For this review, take the finished solid that the model builds, in its own axes (mm). A direction names the side the tool comes from. Coordinates: 2 decimals unless noted, no trailing zeros. Loops run counter-clockwise (first coordinate to the right, second up) from the corner with the lowest first, then second, coordinate; pieces in that order, holes last. Notation, with made-up numbers: (28.25, 87) -> (71.25, 87) arc R13 cw to (71.25, 92) -> close; hole circle Ø9 at (85.5, 73.5). An arc over 180 degrees is marked (long way). One line per item, written item: value.
from build123d import *

# Parameters (mm, degrees)
CROQUIS1_W              = 76.2
CROQUIS1_H              = 76.2
CROQUIS1_W_2            = 66.675
CROQUIS1_H_2            = 66.675
SALIENTE_EXTRUIR1_DEPTH = 950
CORTAR_EXTRUIR1_REACH   = 958.093
CORTAR_EXTRUIR2_DEPTH   = 76.2


with BuildPart() as part:
    # Croquis1 → Saliente-Extruir1 (new body)
    with BuildSketch(Plane(origin=(0, 0, 0), x_dir=(1, 0, 0), z_dir=(0, 1, 0))):
        with Locations((38.1, -38.1)):
            Rectangle(CROQUIS1_W, CROQUIS1_H)
        with Locations((38.1, -38.1)):
            Rectangle(CROQUIS1_W_2, CROQUIS1_H_2, mode=Mode.SUBTRACT)
    extrude(amount=SALIENTE_EXTRUIR1_DEPTH)

    # Cortar-Extruir1: up to this face of the body (flat: up to its plane)
    cortar_extruir1_end = Plane(part.part.faces().sort_by_distance((38.1, 475, 0))[0])
    # Croquis2 → Cortar-Extruir1 (cut, up to the picked face)
    with BuildSketch(Plane.XY.offset(76.2), mode=Mode.PRIVATE) as cortar_extruir1_sk1:
        Polygon((0, 0), (76.2, 17.592156164), (76.2, 0), align=None)
    cortar_extruir1_tool1 = split(extrude(cortar_extruir1_sk1.sketch, amount=-CORTAR_EXTRUIR1_REACH, mode=Mode.PRIVATE), bisect_by=cortar_extruir1_end, keep=Keep.BOTH, mode=Mode.PRIVATE)
    add(cortar_extruir1_tool1.solids().sort_by(Axis((50.8, 5.864052, 76.2), (0, 0, -1)))[0], mode=Mode.SUBTRACT)

    # Croquis3 → Cortar-Extruir2 (cut)
    with BuildSketch(Plane.XY.offset(76.2)):
        Polygon((76.2, 950), (0, 932.407843836), (0, 950), align=None)
    extrude(amount=-CORTAR_EXTRUIR2_DEPTH, mode=Mode.SUBTRACT)


solid = part.part
1. Take a section at B-B, the plane z = 63. Give the boundary of the cut face in (x, y), and give its area (3 significant figures).
Return value:
outline: (0, 0) -> (4.76, 1.1) -> (4.76, 933.51) -> (0, 932.41) -> close; (71.44, 16.49) -> (76.2, 17.59) -> (76.2, 950) -> (71.44, 948.9) -> close
area: 8,880 mm2
2. Insertion check: pin 1 Ø10 at (x, z) = (41, 13) entering from +Y. The pin has a flat end and moves straight along its axis. Give the tip position at first contact, or say it passes through.
Return value:
pin 1: passes through
3. To check wall thickness, follow probe 1 along Z at (x, y) = (55, 141.5); probe 2 along Y at (x, z) = (72, 29). State the ranges of each line that lie inside material, in increasing order. Write a range as from..to.
Return value:
probe 1: z = 0..4.76, 71.44..76.2
probe 2: y = 16.62..949.03
4. For faces 1 (the flat face through (38, 468, 0)), 2 (the flat face through (38, 468, 71.438)), list the 3-axis set-ups (+Z, -Z, +X, -X, +Y, -Y) from which the entire face can be reached by the end or side of a thin tool; tool diameter is ignored.
Return value:
face 1: -Z, +X, -X, +Y, -Y
face 2: +Y, -Y
5. Take a section at C-C, the plane x = 42.5. Give the boundary of the cut face in (y, z).
Return value:
outline: (9.81, 0) -> (942.22, 0) -> (942.22, 4.76) -> (9.81, 4.76) -> close; (9.81, 71.44) -> (942.22, 71.44) -> (942.22, 76.2) -> (9.81, 76.2) -> close
6. The part is to be moulded in two halves that separate along X. For faces 3 (the flat face through (71.438, 476, 39)), 4 (the flat face through (0, 460, 39)), 5 (the flat face through (76.2, 477, 39)), 6 (the flat face through (38, 468, 76.2)), say which applies: pulls with the +X half, pulls with the -X half, needs draft (parallel to the pull), parting line crosses it, or undercut.
Return value:
face 3: undercut
face 4: pulls with the -X half
face 5: pulls with the +X half
face 6: needs draft
7. Take a section at A-A, the plane y = 711.5. Give the boundary of the cut face in (x, z), and give its area (3 significant figures).
Return value:
outline: (0, 0) -> (76.2, 0) -> (76.2, 76.2) -> (0, 76.2) -> close; hole (4.76, 4.76) -> (71.44, 4.76) -> (71.44, 71.44) -> (4.76, 71.44) -> close
area: 1,360 mm2
